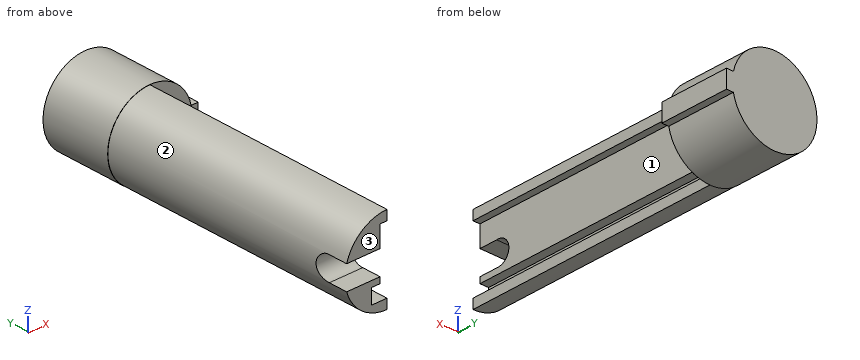
```python
from build123d import *

# Parameters (mm, degrees)
PAD_DEPTH       = 15
POCKET_DEPTH    = 13
PAD001_DEPTH    = 55
POCKET001_DEPTH = 7.601


with BuildPart() as part:
    # Sketch → Pad (new body)
    with BuildSketch(Plane.XZ):
        with BuildLine():
            ThreePointArc((8.889624, 1.945402), (-9.099882, -0.046426), (8.90901, -1.854598))
            Line((10.40901, -1.854598), (8.90901, -1.854598))
            Line((10.40901, 1.945402), (10.40901, -1.854598))
            Line((8.889624, 1.945402), (10.40901, 1.945402))
        make_face()
    extrude(amount=PAD_DEPTH)

    # Sketch001 (on Face6 of Pad) → Pocket (cut)
    with BuildSketch(Plane.XZ.offset(15)):
        Polygon((-1.5, 7), (1.5, 7), (1.5, -7), (-3.348355, -7), (-3.348355, -3.808815), (-1.5, -3.808815), align=None)
    extrude(amount=-POCKET_DEPTH, mode=Mode.SUBTRACT)

    # Sketch002 (on Face5 of Pocket) → Pad001 (join)
    with BuildSketch(Plane.XZ.offset(15)):
        with BuildLine():
            Line((0, 7), (-1.5, 7))
            Line((-1.5, 7), (-1.5, -3.808815))
            Line((-1.5, -3.808815), (-3.348355, -3.808815))
            Line((-3.348355, -3.808815), (-3.348355, -7))
            Line((-3.348355, -7), (0, -7))
            Line((0, -7), (0, -9.054887))
            ThreePointArc((0, 9.054887), (-9.054887, 0), (0, -9.054887))
            Line((0, 7), (0, 9.054887))
        make_face()
    extrude(amount=PAD001_DEPTH)

    # Sketch003 (on Face19 of Pad001) → Pocket001 (cut, through all)
    with BuildSketch(Plane(origin=(-1.5, 0, 0), x_dir=(0, 0, 1), z_dir=(1, 0, 0))):
        with BuildLine():
            Line((-2.546247, 70), (-2.546247, 65.982418))
            ThreePointArc((-2.546247, 65.982418), (0.071035, 63.295116), (2.534594, 66.124008))
            Line((2.534594, 70), (2.534594, 66.124008))
            Line((-2.546247, 70), (2.534594, 70))
        make_face()
    extrude(amount=-POCKET001_DEPTH, mode=Mode.SUBTRACT)


solid = part.part
```
Input: part model. Units: mm. Frame: model coordinates. Face numbers are marked on the shaded views. Round coordinates to 2 decimals unless told otherwise and drop trailing zeros. Loops run counter-clockwise (first coordinate to the right, second up) from the corner with the lowest first, then second, coordinate; pieces in that order, holes last. Notation, with made-up numbers: (28.5, -34.5) -> (46.5, -34.5) arc R19 cw to (46.5, -26.5) -> close; hole circle Ø8 at (-2.75, -11). An arc over 180 degrees is marked (long way). One line per item, written item: value.
(1) Section A-A (y = -57). Return the cut outline in (x, z).
Geometry check:
outline: (-3.35, -7) -> (-3.35, -3.81) -> (-1.5, -3.81) -> (-1.5, 7) -> (0, 7) -> (0, 9.05) arc R9.05 ccw to (0, -9.05) -> (0, -7) -> close
(2) Pin query (flat end, axial travel): pin 1 (1.5 mm diameter, centred on x = 2.5, z = -2, fed in from -Y); pin 2 (1.2 mm diameter, centred on x = -6, y = -68.5, fed in from -Z); pin 3 (0.8 mm diameter, centred on x = 9.5, y = -7, fed in from -Z). Return the tip coordinate at first contact, or that it passes through.
Geometry check:
pin 1: y = -15
pin 2: z = -7.27
pin 3: z = -1.85
(3) Material intervals for line 1 (X direction, y = -3, z = 0.5); line 2 (Y direction, x = -5.75, z = 0); line 3 (Y direction, x = 4.5, z = 4), sorted ascending. Write a range as [from, to].
Geometry check:
line 1: [-9.09, -1.5], [1.5, 10.41]
line 2: [-63.29, 0]
line 3: [-15, 0]
(4) Section D-D (z = -6.25). Return the cut outline in (x, y), plus the area to 3 significant figures.
Geometry check:
outline: (-6.61, -15) -> (-6.55, -15) -> (-6.55, -70) -> (-3.35, -70) -> (-3.35, -2) -> (1.5, -2) -> (1.5, -15) -> (6.61, -15) -> (6.61, 0) -> (-6.61, 0) -> close
area: 312 mm2
(5) Mould query, pull axis X, two halves, no side actions, for the marked faces 1, 2 and 3. Classes: pulls with the +X half, pulls with the -X half, needs draft (parallel to the pull), parting line crosses it, or undercut.
Geometry check:
face 1: undercut
face 2: pulls with the -X half
face 3: needs draft
(6) Section B-B (z = 0). Return the cut outline in (x, y), plus the area to 3 significant figures.
Geometry check:
outline: (-9.1, -15) -> (-9.05, -15) -> (-9.05, -63.29) -> (-1.5, -63.29) -> (-1.5, -2) -> (1.5, -2) -> (1.5, -15) -> (10.41, -15) -> (10.41, 0) -> (-9.1, 0) -> close
area: 618 mm2
(7) Section C-C (x = -8). Return the cut outline in (y, z), plus the area to 3 significant figures.
Geometry check:
outline: (-70, -4.24) -> (-15, -4.24) -> (-15, -4.34) -> (0, -4.34) -> (0, 4.34) -> (-15, 4.34) -> (-15, 4.24) -> (-70, 4.24) -> (-70, 2.53) -> (-66.12, 2.53) arc R2.55 cw (long way) to (-65.98, -2.55) -> (-70, -2.55) -> close
area: 565 mm2
